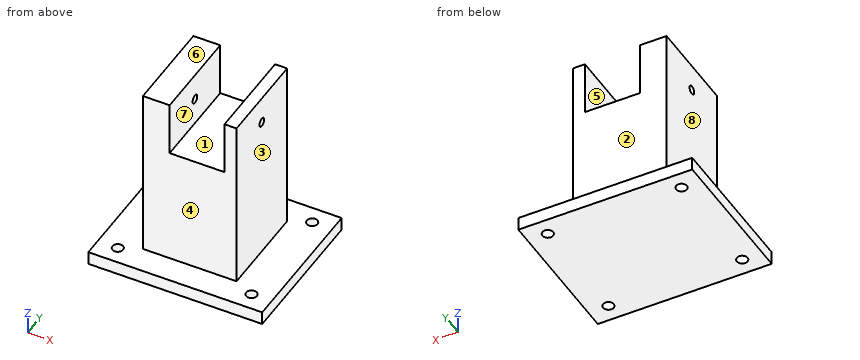
Autodesk Fusion 360 part; units mm, degrees
sketch "Boceto2" plane through (0, 0, 0) normal (0, 0, 1) x (1, 0, 0)
  line L0 (0, 0) -> (35, 0)
  line L1 (35, 0) -> (35, 35)
  line L2 (35, 35) -> (0, 35)
  line L3 (0, 35) -> (0, 0)
  line L4 (50, -10) -> (-15, -10)
  line L5 (-15, -10) -> (-15, 45)
  line L6 (-15, 45) -> (50, 45)
  line L7 (50, 45) -> (50, -10)
  line L8 (50, -10) -> (-15, 45) construction
  line L9 (-15, -10) -> (50, 45) construction
  line L10 (42.5, 38.5) -> (-7.5, 38.5) construction
  line L11 (-7.5, 38.5) -> (-7.5, -3.5) construction
  line L12 (-7.5, -3.5) -> (42.5, -3.5) construction
  line L13 (42.5, -3.5) -> (42.5, 38.5) construction
  line L14 (42.5, 38.5) -> (-7.5, -3.5) construction
  line L15 (-7.5, 38.5) -> (42.5, -3.5) construction
  circle A0 centre (42.5, 38.5) radius 2
  line L16 (17.5, 45) -> (17.5, -10) construction
  line L17 (-15, 17.5) -> (50, 17.5) construction
  circle A1 centre (-7.5, 38.5) radius 2
  circle A2 centre (-7.5, -3.5) radius 2
  circle A3 centre (42.5, -3.5) radius 2
  point P0 (17.5, 17.5)
  point P1 (17.5, 17.5)
  dimension "d8" = 35
  dimension "d9" = 35
  dimension "d10" = 15
  dimension "d12" = 10
  dimension "d13" = 10
  dimension "d14" = 15
  dimension "d15" = 50
  dimension "d16" = 42
  dimension "d17" = 4
extrude "Extruir1" add sketch "Boceto2" along normal blind 70.5 contours L0 L1 L2 L3
sketch "Boceto3" plane through (0, 0, 0) normal (0, -1, 0) x (1, 0, 0)
  line L0 (0, 0) -> (35, 0)
  line L1 (35, 0) -> (35, 70.5)
  line L2 (35, 70.5) -> (0, 70.5)
  line L3 (0, 70.5) -> (0, 0)
  line L4 (0, 70.5) -> (10, 70.5)
  line L5 (10, 70.5) -> (30.5, 70.5)
  line L6 (30.5, 70.5) -> (30.5, 50)
  line L7 (30.5, 50) -> (10, 50)
  line L8 (10, 50) -> (10, 70.5)
  dimension "d3" = 10
  dimension "d4" = 20.5
  dimension "d5" = 20.5
extrude "Extruir2" cut sketch "Boceto3" against normal blind 35 contours L2 L5 L6 L7 L8
sketch "Boceto4" plane through (0, 0, 50) normal (0, 0, 1) x (-1, 0, 0)
  line L0 (-10, 0) -> (-30.5, 0)
  line L1 (-30.5, 0) -> (-30.5, -35)
  line L2 (-30.5, -35) -> (-10, -35)
  line L3 (-10, -35) -> (-10, 0)
  line L4 (-20.25, -35) -> (-20.25, 0)
extrude "Extruir3" add sketch "Boceto2" along normal blind 5
sketch "Boceto5" plane through (35, 0, 0) normal (1, 0, 0) x (0, 1, 0)
  line L0 (0, 5) -> (35, 5)
  line L1 (35, 5) -> (35, 70.5)
  line L2 (35, 70.5) -> (0, 70.5)
  line L3 (0, 70.5) -> (0, 5)
  line L4 (0, 70.5) -> (35, 70.5)
  line L5 (35, 70.5) -> (35, 50)
  line L6 (35, 50) -> (0, 50)
  line L7 (0, 50) -> (0, 70.5)
  circle A0 centre (17.5, 60.25) radius 1.6
  dimension "d20" = 3.2
extrude "Extruir4" cut sketch "Boceto5" against normal blind 45 contours A0
Input: part model. Units: mm. Frame: model coordinates. Face numbers are marked on the shaded views. A direction names the side the tool comes from. Coordinates: 2 decimals unless noted, no trailing zeros. Loops run counter-clockwise (first coordinate to the right, second up) from the corner with the lowest first, then second, coordinate; pieces in that order, holes last.
Q1. Section C-C, the plane x = 43. Return the cut outline in (y, z), and give its area (3 significant figures).
Results are:
outline: (-10, 0) - (-5.44, 0) - (-5.44, 5) - (-10, 5) - close; (-1.56, 0) - (36.56, 0) - (36.56, 5) - (-1.56, 5) - close; (40.44, 0) - (45, 0) - (45, 5) - (40.44, 5) - close
area: 236 mm2
Q2. Mould query, pull axis X, two halves, no side actions, for the marked faces 5, 6, 7 and 8. Classes: +X half, -X half, draft (parallel to the pull), parting line (faces both ways), or undercut.
Results are:
face 5: undercut
face 6: draft
face 7: undercut
face 8: -X half
Q3. Contact query for flat-ended pins moving along their axis: pin 1 (16.5 mm diameter, centred on y = 11, z = 60.5, fed in from +X); pin 2 (5 mm diameter, centred on x = 7, z = 34.5, fed in from -Y); pin 3 (1 mm diameter, centred on y = 5.5, z = 40.5, fed in from -X). Output: stop coordinate, or through.
Results are:
pin 1: stops at x = 35
pin 2: stops at y = 0
pin 3: stops at x = 0
Q4. Line query: line 1 along Y through (x, z) = (-7.5, 3.7); line 2 along X through (y, z) = (29, 61); line 3 along Z through (x, y) = (32.65, 17.5). Output: solid intervals per line, ascending.
Results are:
line 1: y = -10 to -5.5, -1.5 to 36.5, 40.5 to 45
line 2: x = 0 to 10, 30.5 to 35
line 3: z = 0 to 58.65, 61.85 to 70.5
Q5. Section B-B, the plane z = 60.25. Return the cut outline in (x, y).
Results are:
outline: (0, 0) - (10, 0) - (10, 15.9) - (0, 15.9) - close; (0, 19.1) - (10, 19.1) - (10, 35) - (0, 35) - close; (30.5, 0) - (35, 0) - (35, 15.9) - (30.5, 15.9) - close; (30.5, 19.1) - (35, 19.1) - (35, 35) - (30.5, 35) - close
Q6. Set-up query: the marked faces 1, 2, 3 and 4. Return all of +Z, -Z, +X, -X, +Y, -Y with unobstructed straight access to the full face (end or side cutting, diameter ignored); none if empty.
Results are:
face 1: +Z, +Y, -Y
face 2: +Z, +X, -X, +Y
face 3: +Z, +X, +Y, -Y
face 4: +Z, +X, -X, -Y
Q7. Section A-A, the plane y = 17.5. Return the cut outline in (x, z), and give its area (3 significant figures).
Results are:
outline: (-15, 0) - (50, 0) - (50, 5) - (35, 5) - (35, 58.65) - (30.5, 58.65) - (30.5, 50) - (10, 50) - (10, 58.65) - (0, 58.65) - (0, 5) - (-15, 5) - close; (0, 61.85) - (10, 61.85) - (10, 70.5) - (0, 70.5) - close; (30.5, 61.85) - (35, 61.85) - (35, 70.5) - (30.5, 70.5) - close
area: 2,150 mm2
Q8. Section D-D, the plane y = -3.5. Return the cut outline in (x, z).
Results are:
outline: (-15, 0) - (-9.5, 0) - (-9.5, 5) - (-15, 5) - close; (-5.5, 0) - (40.5, 0) - (40.5, 5) - (-5.5, 5) - close; (44.5, 0) - (50, 0) - (50, 5) - (44.5, 5) - close
